from build123d import *

# Parameters (mm, degrees)
ESBO_O1_R                = 2
ESBO_O1_R_2              = 1.25
RESSALTO_EXTRUS_O1_DEPTH = 3
CORTE_EXTRUS_O1_START    = -4
ESBO_O6_R                = 1.4
CORTE_EXTRUS_O1_DEPTH    = 5


with BuildPart() as part:
    # Esboço1 → Ressalto-extrusão1 (new body)
    with BuildSketch(Plane.XY):
        with BuildLine():
            Line((6.614378278, 2.5), (30, 2.5))
            ThreePointArc((30, 2.5), (31.767766953, 1.767766953), (32.5, 0))
            ThreePointArc((32.5, 0), (31.767766953, -1.767766953), (30, -2.5))
            Line((30, -2.5), (6.614378278, -2.5))
            ThreePointArc((6.614378278, -2.5), (5.678963931, -2.732233047), (4.960783708, -3.375))
            ThreePointArc((4.960783708, -3.375), (0, -6), (-4.960783708, -3.375))
            ThreePointArc((-4.960783708, -3.375), (-5.678963931, -2.732233047), (-6.614378278, -2.5))
            Line((-6.614378278, -2.5), (-30, -2.5))
            ThreePointArc((-30, -2.5), (-31.767766953, -1.767766953), (-32.5, 0))
            ThreePointArc((-32.5, 0), (-31.767766953, 1.767766953), (-30, 2.5))
            Line((-30, 2.5), (-6.614378278, 2.5))
            ThreePointArc((-6.614378278, 2.5), (-5.678963931, 2.732233047), (-4.960783708, 3.375))
            ThreePointArc((-4.960783708, 3.375), (0, 6), (4.960783708, 3.375))
            ThreePointArc((4.960783708, 3.375), (5.678963931, 2.732233047), (6.614378278, 2.5))
        make_face()
        Circle(ESBO_O1_R, mode=Mode.SUBTRACT)
        with Locations((10, 0)):
            Circle(ESBO_O1_R_2, mode=Mode.SUBTRACT)
    extrude(amount=RESSALTO_EXTRUS_O1_DEPTH)

    # Esboço6 → Corte-extrusão1 (cut)
    with BuildSketch(Plane(origin=(0, 0, 3), x_dir=(0, 1, 0), z_dir=(0, 0, 1)).offset(CORTE_EXTRUS_O1_START)):
        with Locations((0, 30)):
            Circle(ESBO_O6_R)
    corte_extrus_o1 = extrude(amount=CORTE_EXTRUS_O1_DEPTH, mode=Mode.SUBTRACT)

    # Espelhar1: Corte-extrusão1 across plane
    add(corte_extrus_o1.mirror(Plane(origin=(0, 0, 0), x_dir=(0, 0, 1), z_dir=(1, 0, 0))), mode=Mode.SUBTRACT)


solid = part.part
Here's how the part is built. I have some questions about the finished solid (model axes, mm). A direction names the side the tool comes from. Give positions to 0.01 mm unless a question says otherwise; leave off trailing zeros. Order: outer loops, then holes, each group sorted by start corner. A loop starts at its lowest first (then second) coordinate and runs counter-clockwise, first axis right, second up. Notation, with made-up numbers: (-8.75, 73.5) -> (6.25, 73.5) arc R23 ccw to (6.25, 93.5) -> close; hole circle Ø7 at (56, 61). An arc over 180 degrees is marked (long way). Use a Markdown table: item, result. Add a question column.
Item 1: Imagine slicing it at D-D on x = -8. Please give me the cut outline in (y, z).
Item 2: Imagine slicing it at C-C on x = 10. Please give me the cut outline in (y, z).
Item 3: I need wall thicknesses on line 1 (Y direction, x = 10, z = 2.1); line 2 (Y direction, x = 20, z = 2.7); line 3 (X direction, y = -1.5, z = 1.5). Which ranges of each line are inside material? Lowest first, please.
Item 4: Imagine slicing it at B-B on z = 2.35. Please give me the cut outline in (x, y) (3 decimals), plus the area to 3 significant figures.
Item 5: Will these pins go through, and if not, where does the flat tip stop? pin 1 (2.5 mm diameter, centred on x = -30, y = 0, fed in from -Z); pin 2 (1.5 mm diameter, centred on x = 18.5, z = 1.5, fed in from +Y).
Item 6: For faces 4 (the face through (18, 2.5, 1)), 5 (the face through (-18, -2.5, 1)), 6 (the face through (-18, 2.5, 1)), which set-ups out of +Z, -Z, +X, -X, +Y, -Y let a thin tool reach every point of the face, with its end or its side?
Item 7: Imagine slicing it at A-A on x = 0. Please give me the cut outline in (y, z), plus the area to 3 significant figures.
Item 8: If we mould it in two halves opening along Y, with no side actions, what happens to faces 1 (the face through (0, -6, 1)), 2 (the face through (8.75, 0.05, 1.48)), 3 (the face through (3, 0, 0))? For each: pulls with the +Y half, pulls with the -Y half, needs draft (parallel to the pull), parting line crosses it, or undercut.
Data:
| question | item | result |
|---|---|---|
| 1 | outline | (-2.5, 0) -> (2.5, 0) -> (2.5, 3) -> (-2.5, 3) -> close |
| 2 | outline | (-2.5, 0) -> (-1.25, 0) -> (-1.25, 3) -> (-2.5, 3) -> close; (1.25, 0) -> (2.5, 0) -> (2.5, 3) -> (1.25, 3) -> close |
| 3 | line 1 | y = -2.5 to -1.25, 1.25 to 2.5 |
| 3 | line 2 | y = -2.5 to 2.5 |
| 3 | line 3 | x = -32 to -1.32, 1.32 to 32 |
| 4 | outline | (-30, -2.5) -> (-6.614, -2.5) arc R2 cw to (-4.961, -3.375) arc R6 ccw to (4.961, -3.375) arc R2 cw to (6.614, -2.5) -> (30, -2.5) arc R2.5 ccw to (30, 2.5) -> (6.614, 2.5) arc R2 cw to (4.961, 3.375) arc R6 ccw to (-4.961, 3.375) arc R2 cw to (-6.614, 2.5) -> (-30, 2.5) arc R2.5 ccw to start; hole circle Ø2.8 at (-30, 0); hole circle Ø4 at (0, 0); hole circle Ø2.5 at (10, 0); hole circle Ø2.8 at (30, 0) |
| 4 | area | 346 mm² |
| 5 | pin 1 | passes through |
| 5 | pin 2 | stops at y = 2.5 |
| 6 | face 4 | +Z, -Z, +X, +Y |
| 6 | face 5 | +Z, -Z, -X, -Y |
| 6 | face 6 | +Z, -Z, -X, +Y |
| 7 | outline | (-6, 0) -> (-2, 0) -> (-2, 3) -> (-6, 3) -> close; (2, 0) -> (6, 0) -> (6, 3) -> (2, 3) -> close |
| 7 | area | 24.0 mm² |
| 8 | face 1 | pulls with the -Y half |
| 8 | face 2 | undercut |
| 8 | face 3 | needs draft |
